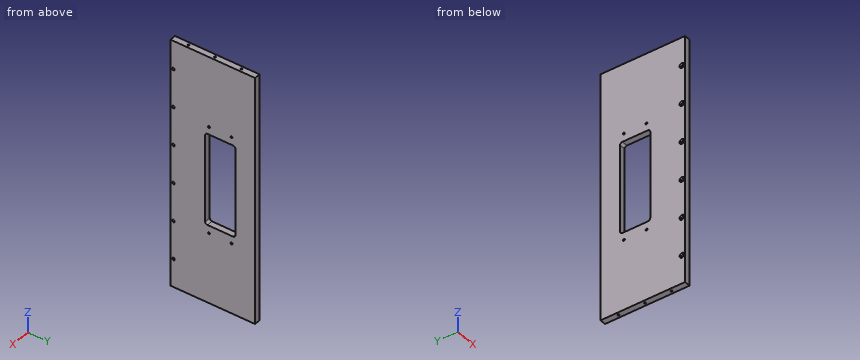
```python
from build123d import *

# Parameters (mm, degrees)
SKETCH1_W                                     = 324
SKETCH1_H                                     = 112
BOSS_EXTRUDE1_DEPTH                           = 8
M3X0_5_TAPPED_HOLE1_AT_2_COUNT                = 2
M3X0_5_TAPPED_HOLE1_AT_2_PITCH                = 35
M3X0_5_TAPPED_HOLE1_AT_3_COUNT                = 2
M3X0_5_TAPPED_HOLE1_AT_3_PITCH                = 70
CSK_FOR_M3_COUNTERSUNK_FLAT_HEAD1_D           = 3.4
CSK_FOR_M3_COUNTERSUNK_FLAT_HEAD1_DEPTH       = 11.5
CSK_FOR_M3_COUNTERSUNK_FLAT_HEAD1_CSINK_D     = 6.3
CSK_FOR_M3_COUNTERSUNK_FLAT_HEAD1_CSINK_ANGLE = 90
CSK_FOR_M3_COUNTERSUNK_FLAT_HEAD1_TIP         = 1.021463052
SKETCH9_W                                     = 120
SKETCH9_H                                     = 40
CUT_EXTRUDE1_DEPTH                            = 172.59254063
M3X0_5_TAPPED_HOLE2_D                         = 2.5
FILLET1_R                                     = 3


with BuildPart() as part:
    # Sketch1 → Boss-Extrude1 (new body)
    with BuildSketch(Plane(origin=(0, 0, 0), x_dir=(0, 0, -1), z_dir=(1, 0, 0))):
        Rectangle(SKETCH1_W, SKETCH1_H)
    extrude(amount=BOSS_EXTRUDE1_DEPTH)

    # Sketch4 → M3x0.5 Tapped Hole1 (revolve, cut)
    with BuildSketch(Plane(origin=(4, 35, 162), x_dir=(0, -1, 0), z_dir=(1, 0, 0))):
        Polygon((0, 0), (0, 12.251075774), (1.25, 11.5), (1.25, 0), align=None)
    m3x0_5_tapped_hole1 = revolve(axis=Axis((4, 35, 168.35), (0, 0, -1)), mode=Mode.SUBTRACT)

    # M3x0.5 Tapped Hole1 at 2: M3x0.5 Tapped Hole1 ×2
    with Locations(*[(0, -i * M3X0_5_TAPPED_HOLE1_AT_2_PITCH, 0) for i in range(1, M3X0_5_TAPPED_HOLE1_AT_2_COUNT)]):
        add(m3x0_5_tapped_hole1, mode=Mode.SUBTRACT)

    # M3x0.5 Tapped Hole1 at 3: M3x0.5 Tapped Hole1 ×2
    with Locations(*[(0, -i * M3X0_5_TAPPED_HOLE1_AT_3_PITCH, 0) for i in range(1, M3X0_5_TAPPED_HOLE1_AT_3_COUNT)]):
        add(m3x0_5_tapped_hole1, mode=Mode.SUBTRACT)

    # Mirror1: M3x0.5 Tapped Hole1 across plane
    add(m3x0_5_tapped_hole1.mirror(Plane.XY), mode=Mode.SUBTRACT)

    # Mirror1 copy 1 sketch → Mirror1 copy 1 (revolve, cut)
    with BuildSketch(Plane(origin=(4, 0, -162), x_dir=(0, -1, 0), z_dir=(1, 0, 0))):
        Polygon((0, 0), (0, -12.251075774), (1.25, -11.5), (1.25, 0), align=None)
    revolve(axis=Axis((4, 0, -168.35), (0, 0, -1)), mode=Mode.SUBTRACT)

    # Mirror1 copy 2 sketch → Mirror1 copy 2 (revolve, cut)
    with BuildSketch(Plane(origin=(4, -35, -162), x_dir=(0, -1, 0), z_dir=(1, 0, 0))):
        Polygon((0, 0), (0, -12.251075774), (1.25, -11.5), (1.25, 0), align=None)
    revolve(axis=Axis((4, -35, -168.35), (0, 0, -1)), mode=Mode.SUBTRACT)

    # CSK for M3 Countersunk Flat Head1
    with Locations(Plane(origin=(0, -52, -125), x_dir=(0, 0, -1), z_dir=(-1, 0, 0))):
        with Locations((0, 0), (-50, 0), (-100, 0), (-150, 0), (-200, 0), (-250, 0)):
            CounterSinkHole(CSK_FOR_M3_COUNTERSUNK_FLAT_HEAD1_D / 2, CSK_FOR_M3_COUNTERSUNK_FLAT_HEAD1_CSINK_D / 2, depth=CSK_FOR_M3_COUNTERSUNK_FLAT_HEAD1_DEPTH, counter_sink_angle=CSK_FOR_M3_COUNTERSUNK_FLAT_HEAD1_CSINK_ANGLE)
            with Locations((0, 0, -(CSK_FOR_M3_COUNTERSUNK_FLAT_HEAD1_DEPTH + CSK_FOR_M3_COUNTERSUNK_FLAT_HEAD1_TIP / 2))):  # 118° drill point
                Cone(0, CSK_FOR_M3_COUNTERSUNK_FLAT_HEAD1_D / 2, CSK_FOR_M3_COUNTERSUNK_FLAT_HEAD1_TIP, mode=Mode.SUBTRACT)

    # Sketch9 → Cut-Extrude1 (cut, through all)
    with BuildSketch(Plane.ZY):
        with Locations((0, 10)):
            Rectangle(SKETCH9_W, SKETCH9_H)
    extrude(amount=-CUT_EXTRUDE1_DEPTH, mode=Mode.SUBTRACT)

    # M3x0.5 Tapped Hole2 (through all)
    with Locations(Plane(origin=(0, 25, -70), x_dir=(0, 0, -1), z_dir=(-1, 0, 0))):
        with Locations((0, 0), (0, 30)):
            m3x0_5_tapped_hole2 = Hole(M3X0_5_TAPPED_HOLE2_D / 2)

    # Mirror2: M3x0.5 Tapped Hole2 across plane
    add(m3x0_5_tapped_hole2.mirror(Plane.XY), mode=Mode.SUBTRACT)

    # Fillet1
    fillet1_edges = [part.edges().sort_by_distance(p)[0] for p in [
        (4, -10, -60),
        (4, 30, -60),
        (4, 30, 60),
        (4, -10, 60),
    ]]
    fillet(fillet1_edges, radius=FILLET1_R)


solid = part.part
```
The model under review builds one solid part; all positions refer to its coordinate system, in mm. Coordinates: 2 decimals unless noted, no trailing zeros. Order: outer loops, then holes, each group sorted by start corner. A loop starts at its lowest first (then second) coordinate and runs counter-clockwise, first axis right, second up. Notation, with made-up numbers: (36, 88.25) -> (45, 88.25) arc R31 cw to (45, 122.25) -> close; hole circle Ø5 at (45, 42.5). An arc over 180 degrees is marked (long way). Answer in a Markdown table with one row per item. Add a question column.
Item 1: We need section B-B on y = 13.5. Write out the cut boundary in (x, z), plus the area to 3 significant figures.
Item 2: We need section A-A on z = -42. Write out the cut boundary in (x, y), plus the area to 3 significant figures.
Item 3: Clearance check with flat-ended pins moving along their axes: pin 1 (3 mm diameter, centred on x = 4, y = 35, fed in from -Z); pin 2 (2 mm diameter, centred on x = 4, y = 0, fed in from -Z). State where each tip first meets the part, or that it passes through.
Item 4: To check wall thickness, follow probe 1 along Y at (x, z) = (5, 70); probe 2 along Y at (x, z) = (4, 156); probe 3 along Y at (x, z) = (4.75, -25). State the ranges of each line that lie inside material, in increasing order.
Final values:
| question | item | result |
|---|---|---|
| 1 | outline | (0, -162) -> (8, -162) -> (8, -60) -> (0, -60) -> close; (0, 60) -> (8, 60) -> (8, 162) -> (0, 162) -> close |
| 1 | area | 1,630 mm2 |
| 2 | outline | (0, -56) -> (8, -56) -> (8, -10) -> (0, -10) -> close; (0, 30) -> (8, 30) -> (8, 56) -> (0, 56) -> close |
| 2 | area | 576 mm2 |
| 3 | pin 1 | stops at z = -162 |
| 3 | pin 2 | stops at z = -150.35 |
| 4 | probe 1 | y = -56 to -6.25, -3.75 to 23.75, 26.25 to 56 |
| 4 | probe 2 | y = -56 to -36.25, -33.75 to -1.25, 1.25 to 33.75, 36.25 to 56 |
| 4 | probe 3 | y = -56 to -53.7, -50.3 to -10, 30 to 56 |
